```python
from build123d import *

# Parameters (mm, degrees)
BOSS_EXTRUDE1_DEPTH = 50.8
CUT_EXTRUDE4_DEPTH  = 73.955945611


with BuildPart() as part:
    # Sketch1 → Boss-Extrude1 (new body)
    with BuildSketch(Plane.XY):
        Polygon((-9.525, -22.225), (12.7, -22.225), (12.7, -25.4), (-12.7, -25.4), (-12.7, 25.4), (-9.525, 25.4), align=None)
    extrude(amount=BOSS_EXTRUDE1_DEPTH)

    # Sketch6 → Cut-Extrude4 (cut, through all)
    with BuildSketch(Plane.XZ.offset(25.4)):
        Polygon((-12.7, 0), (12.7, 25.4), (12.7, 0), align=None)
    extrude(amount=-CUT_EXTRUDE4_DEPTH, mode=Mode.SUBTRACT)


solid = part.part
```
CAD build for the part. Positions are in the model's coordinates, mm. A direction names the side the tool comes from. Round coordinates to 2 decimals unless told otherwise and drop trailing zeros. Order: outer loops, then holes, each group sorted by start corner. A loop starts at its lowest first (then second) coordinate and runs counter-clockwise, first axis right, second up.
Item 1: Saw through at B-B on x = 11.25. Write the cut outline in (y, z) (3 decimals).
Item 2: Tool access for faces 1 (the face through (-12.7, 0, 25)), 2 (the face through (1, -22.225, 32)): list every direction of +Z, -Z, +X, -X, +Y, -Y with a clear straight run to the whole face (end or side of a thin tool).
Item 3: Pin check, flat tips, straight feed: pin 1 (4 mm diameter, centred on y = 3, z = 13, fed in from +X) (3 decimals); pin 2 (10 mm diameter, centred on x = 0.5, z = 10, fed in from +Y) (3 decimals). Stop position of each tip, or through.
Item 4: Probe line 1 along Y through (x, z) = (-4, 35.5) (3 decimals); line 2 along X through (y, z) = (21, 36.5) (3 decimals). List the from-to ranges inside material, lowest first.
Item 5: Saw through at C-C on y = -0.5. Write the cut outline in (x, z) (3 decimals).
Item 6: Saw through at D-D on z = 24.5. Write the cut outline in (x, y) (3 decimals), then the cut area to 3 significant figures.
Item 7: Saw through at A-A on z = 18.5. Write the cut outline in (x, y) (3 decimals).
Reported:
1. outline: (-25.4, 23.95) - (-22.225, 23.95) - (-22.225, 50.8) - (-25.4, 50.8) - close
2. face 1: +Z, -Z, -X, +Y, -Y
2. face 2: +Z, -Z, +X, +Y
3. pin 1: stops at x = -9.525
3. pin 2: stops at y = -22.225
4. line 1: y = -25.4 to -22.225
4. line 2: x = -12.7 to -9.525
5. outline: (-12.7, 0) - (-9.525, 3.175) - (-9.525, 50.8) - (-12.7, 50.8) - close
6. outline: (-12.7, -25.4) - (11.8, -25.4) - (11.8, -22.225) - (-9.525, -22.225) - (-9.525, 25.4) - (-12.7, 25.4) - close
6. area: 229 mm2
7. outline: (-12.7, -25.4) - (5.8, -25.4) - (5.8, -22.225) - (-9.525, -22.225) - (-9.525, 25.4) - (-12.7, 25.4) - close
